from build123d import *

# Parameters (mm, degrees)
F0_R          = 38.1
F1_DEPTH      = 25.4
F2_R          = 12.7
F3_DEPTH      = 25.401
F5_DEPTH      = 38.101
F5_DEPTH_BACK = 38.101


with BuildPart() as f1:
    # F0 (on Front) → F1 (new body)
    with BuildSketch(Plane.XZ):
        Circle(F0_R)
    extrude(amount=F1_DEPTH)

    # F2 (on face) → F3 (cut, through all)
    with BuildSketch(Plane.XZ.offset(25.4)):
        Circle(F2_R)
    extrude(amount=-F3_DEPTH, mode=Mode.SUBTRACT)

    # F4 (on Top) → F5 (cut, two sides)
    with BuildSketch(Plane.XY) as f5_sk:
        with BuildLine():
            Line((32.0281813408, 0), (-32.0281813408, 0))
            ThreePointArc((-32.0281813408, 0), (0, -3.81), (32.0281813408, 0))
        make_face()
    extrude(amount=-F5_DEPTH, mode=Mode.SUBTRACT)
    extrude(f5_sk.sketch, amount=F5_DEPTH_BACK, mode=Mode.SUBTRACT)


solid = f1.part
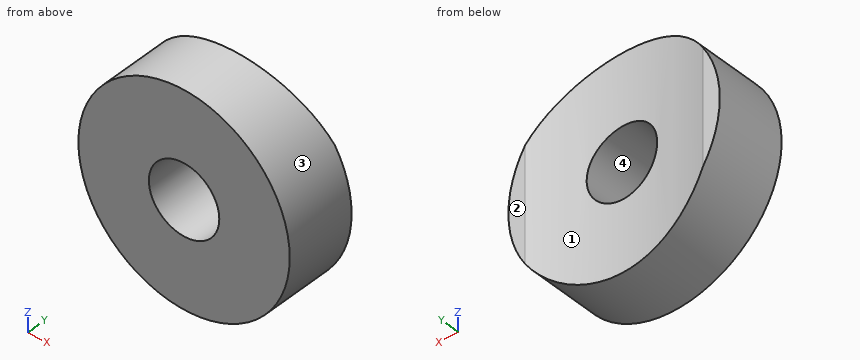
Read the model definition and answer for the solid it produces. Units are mm, in the model's axes. Face numbers are marked on the shaded views. Coordinates: 2 decimals unless noted, no trailing zeros. Order: outer loops, then holes, each group sorted by start corner. A loop starts at its lowest first (then second) coordinate and runs counter-clockwise, first axis right, second up. Notation, with made-up numbers: (25, 35.5) -> (29, 35.5) arc R10 cw to (29, 41.5) -> close; hole circle Ø6 at (-34.5, 46.5). An arc over 180 degrees is marked (long way). Answer as a JSON object with one key per item and string values.
1) A cutting plane is placed at C-C, the plane y = -15.5. Determine the outline of the cut face in (x, z).
Model answer:
{"outline": "circle Ø76.2 at (0, 0); hole circle Ø25.4 at (0, 0)"}
2) The mould has two halves that part along X. Classify the marked faces 1, 2, 3 and 4: released by +X, released by -X, zero draft, split by the parting line, or undercut.
Model answer:
{"face 1": "undercut", "face 2": "zero draft", "face 3": "split by the parting line", "face 4": "undercut"}
3) A cutting plane is placed at B-B, the plane x = 4. Determine the outline of the cut face in (y, z).
Model answer:
{"outline": "(-25.4, -37.89) -> (-3.75, -37.89) -> (-3.75, -12.05) -> (-25.4, -12.05) -> close; (-25.4, 12.05) -> (-3.75, 12.05) -> (-3.75, 37.89) -> (-25.4, 37.89) -> close"}
4) Consider line 1 along Z through (x, y) = (0, -10.5); line 2 along Z through (x, y) = (-8, -10.75). Determine where each line is inside the solid, lowest interval first. Write a range as from..to.
Model answer:
{"line 1": "z = -38.1..-12.7, 12.7..38.1", "line 2": "z = -37.25..-9.86, 9.86..37.25"}
5) A cutting plane is placed at D-D, the plane x = -8. Determine the outline of the cut face in (y, z), plus the area to 3 significant figures.
Model answer:
{"outline": "(-25.4, -37.25) -> (-3.58, -37.25) -> (-3.58, -9.86) -> (-25.4, -9.86) -> close; (-25.4, 9.86) -> (-3.58, 9.86) -> (-3.58, 37.25) -> (-25.4, 37.25) -> close", "area": "1,200 mm²"}
6) A cutting plane is placed at A-A, the plane z = 0. Determine the outline of the cut face in (x, y) (3 decimals), plus the area to 3 significant figures.
Model answer:
{"outline": "(-38.1, -25.4) -> (-12.7, -25.4) -> (-12.7, -3.218) arc R136.525 cw to (-32.028, 0) -> (-38.1, 0) -> close; (12.7, -25.4) -> (38.1, -25.4) -> (38.1, 0) -> (32.028, 0) arc R136.525 cw to (12.7, -3.218) -> close", "area": "1,220 mm²"}
7) Each of these flat-tipped pins is pushed along its axis until it touches: pin 1 (8 mm diameter, centred on x = -6.5, z = -18.5, fed in from +Y); pin 2 (3 mm diameter, centred on y = -22, z = 15, fed in from -X); pin 3 (2 mm diameter, centred on x = 11.5, z = 24.5, fed in from +Y). Where does it stop, or does it pass through?
Model answer:
{"pin 1": "stops at y = -3.41", "pin 2": "stops at x = -35.63", "pin 3": "stops at y = -3.24"}
